from build123d import *

# Parameters (mm, degrees)
SKETCH1_R           = 6.35
SKETCH1_R_2         = 2.54
BOSS_EXTRUDE1_DEPTH = 63.5
SKETCH2_R           = 9.525
SKETCH2_R_2         = 2.54
BOSS_EXTRUDE2_DEPTH = 7.62
CHAMFER1_SIZE       = 7.85840076
CHAMFER1_SIZE_2     = 3.175
FILLET1_R           = 12.7
BOSS_EXTRUDE3_START = -7.62
SKETCH3_R           = 9.525
SKETCH3_R_2         = 2.54
BOSS_EXTRUDE3_DEPTH = 7.62
CHAMFER2_SIZE       = 3.175
CHAMFER2_SIZE_2     = 7.85840076
FILLET2_R           = 12.7
CUT_EXTRUDE1_START  = 6.35
SKETCH4_W           = 29.198575266
SKETCH4_H           = 42.680388974
CUT_EXTRUDE1_DEPTH  = 59.53489827


with BuildPart() as part:
    # Sketch1 → Boss-Extrude1 (new body)
    with BuildSketch(Plane(origin=(0, 0, 0), x_dir=(1, 0, 0), z_dir=(0, 1, 0))):
        with Locations(Location((0, 0, 0), (0, 0, 270))):
            Circle(SKETCH1_R)
        with Locations(Location((0, 0, 0), (0, 0, 270))):
            Circle(SKETCH1_R_2, mode=Mode.SUBTRACT)
    extrude(amount=BOSS_EXTRUDE1_DEPTH)

    # Sketch2 → Boss-Extrude2 (add)
    with BuildSketch(Plane(origin=(0, 0, 0), x_dir=(-1, 0, 0), z_dir=(0, -1, 0))):
        with Locations(Location((0, 0, 0), (0, 0, 90))):
            Circle(SKETCH2_R)
        with Locations(Location((0, 0, 0), (0, 0, 270))):
            Circle(SKETCH2_R_2, mode=Mode.SUBTRACT)
    extrude(amount=-BOSS_EXTRUDE2_DEPTH)

    # Chamfer1
    # the kernel refuses this chamfer: 7.85840076, 3.175 mm, written as the material it takes off along each edge
    with BuildSketch(Plane(origin=(0, 7.62, 0), x_dir=(0, 0, -1), z_dir=(-1, 0, 0))) as chamfer1_piece_1:
        Polygon((9.525, CHAMFER1_SIZE), (9.525 - CHAMFER1_SIZE_2, 0), (9.525, 0), align=None)
    revolve(axis=Axis((0, 7.62, 0), (0, -1, 0)), mode=Mode.SUBTRACT)

    # Fillet1
    fillet1_edges = [part.edges().sort_by_distance(p)[0] for p in [
        (6.35, 7.62, 0),
    ]]
    fillet(fillet1_edges, radius=FILLET1_R)

    # Sketch3 → Boss-Extrude3 (add)
    with BuildSketch(Plane(origin=(0, 63.5, 0), x_dir=(1, 0, 0), z_dir=(0, 1, 0)).offset(BOSS_EXTRUDE3_START)):
        with Locations(Location((0, 0, 0), (0, 0, 270))):
            Circle(SKETCH3_R)
        with Locations(Location((0, 0, 0), (0, 0, 270))):
            Circle(SKETCH3_R_2, mode=Mode.SUBTRACT)
    extrude(amount=BOSS_EXTRUDE3_DEPTH)

    # Chamfer2
    # the kernel refuses this chamfer: 7.85840076, 3.175 mm, written as the material it takes off along each edge
    with BuildSketch(Plane(origin=(0, 55.88, 0), x_dir=(0, 0, 1), z_dir=(-1, 0, 0))) as chamfer2_piece_1_section:
        Polygon((9.525 - CHAMFER2_SIZE, 0), (9.525, CHAMFER2_SIZE_2), (9.525, 0), align=None)
    chamfer2_piece_1 = revolve(axis=Axis((0, 55.88, 0), (0, 1, 0)), mode=Mode.PRIVATE)
    chamfer2_piece_1 = chamfer2_piece_1 - Plane(origin=(0, 59.920436712, 0), x_dir=(0, 0, 1), z_dir=(0, -1, 0)) * Cylinder(6.35, 39, mode=Mode.PRIVATE)
    add(chamfer2_piece_1, mode=Mode.SUBTRACT)

    # Fillet2
    fillet2_edges = [part.edges().sort_by_distance(p)[0] for p in [
        (0, 55.88, -6.35),
    ]]
    fillet(fillet2_edges, radius=FILLET2_R)

    # Sketch4 → Cut-Extrude1 (cut, through all)
    with BuildSketch(Plane.XY.offset(CUT_EXTRUDE1_START)):
        with Locations((0, 16.627867716)):
            Rectangle(SKETCH4_W, SKETCH4_H)
    extrude(amount=CUT_EXTRUDE1_DEPTH, mode=Mode.SUBTRACT)


solid = part.part
Work out the finished part from the listing and answer in its coordinate system (mm). A direction names the side the tool comes from. Give positions to 0.01 mm unless a question says otherwise; leave off trailing zeros. Loops run counter-clockwise (first coordinate to the right, second up) from the corner with the lowest first, then second, coordinate; pieces in that order, holes last. Notation, with made-up numbers: (45.25, 62.5) -> (84.25, 62.5) arc R22 ccw to (84.25, 79.5) -> close; hole circle Ø6 at (14.25, 88). An arc over 180 degrees is marked (long way). Use a Markdown table: item, result. Add a question column.
1. Find the intervals of material crossed by probe 1 along X at (y, z) = (47, 0); probe 2 along Y at (x, z) = (-2.25, -8.25); probe 3 along Z at (x, y) = (-0.75, 4), in increasing order.
2. For faces 1 (the flat face through (0, 0, -3)), 2 (the conical face through (-0.272, 5.072, -7.374)), 3 (the flat face through (0, 4, 6.35)), determine the directions among +Z, -Z, +X, -X, +Y, -Y from which every point of the face is accessible in a straight line to the end or side of a thin tool.
3. Determine the mould class of faces 4 (the conical face through (2.226, 58.502, 7.067)), 5 (the flat face through (-2, 63.5, 2)), 6 (the cylindrical face through (2.52, 31.31, -0.33)) for opening direction Z: released by +Z, released by -Z, zero draft, split by the parting line, or undercut.
4. Section A-A on y = 13 is taken. Determine the outline of the cut face in (x, z), and give its area (3 significant figures).
5. Flat-ended cylindrical pins translate along their axes: pin 1 Ø5 at (x, y) = (2, 5.5) entering from +Z; pin 2 Ø6 at (y, z) = (37.5, 6.5) entering from -X; pin 3 Ø6 at (y, z) = (36.5, -0.5) entering from -X. Find the tip coordinate at first contact, or state that the pin passes through.
Results below:
| question | item | result |
|---|---|---|
| 1 | probe 1 | x = -6.35 to -2.54, 2.54 to 6.35 |
| 1 | probe 2 | y = 0 to 2.17, 61.33 to 63.5 |
| 1 | probe 3 | z = -7.78 to -2.43, 2.43 to 6.35 |
| 2 | face 1 | +Z, -Z, +X, -X, -Y |
| 2 | face 2 | none |
| 2 | face 3 | +Z, +X, -X, -Y |
| 3 | face 4 | split by the parting line |
| 3 | face 5 | zero draft |
| 3 | face 6 | undercut |
| 4 | outline | circle Ø12.7 at (0, 0); hole circle Ø5.08 at (0, 0) |
| 4 | area | 106 mm^2 |
| 5 | pin 1 | stops at z = 6.35 |
| 5 | pin 2 | stops at x = -5.3 |
| 5 | pin 3 | stops at x = -6.35 |
